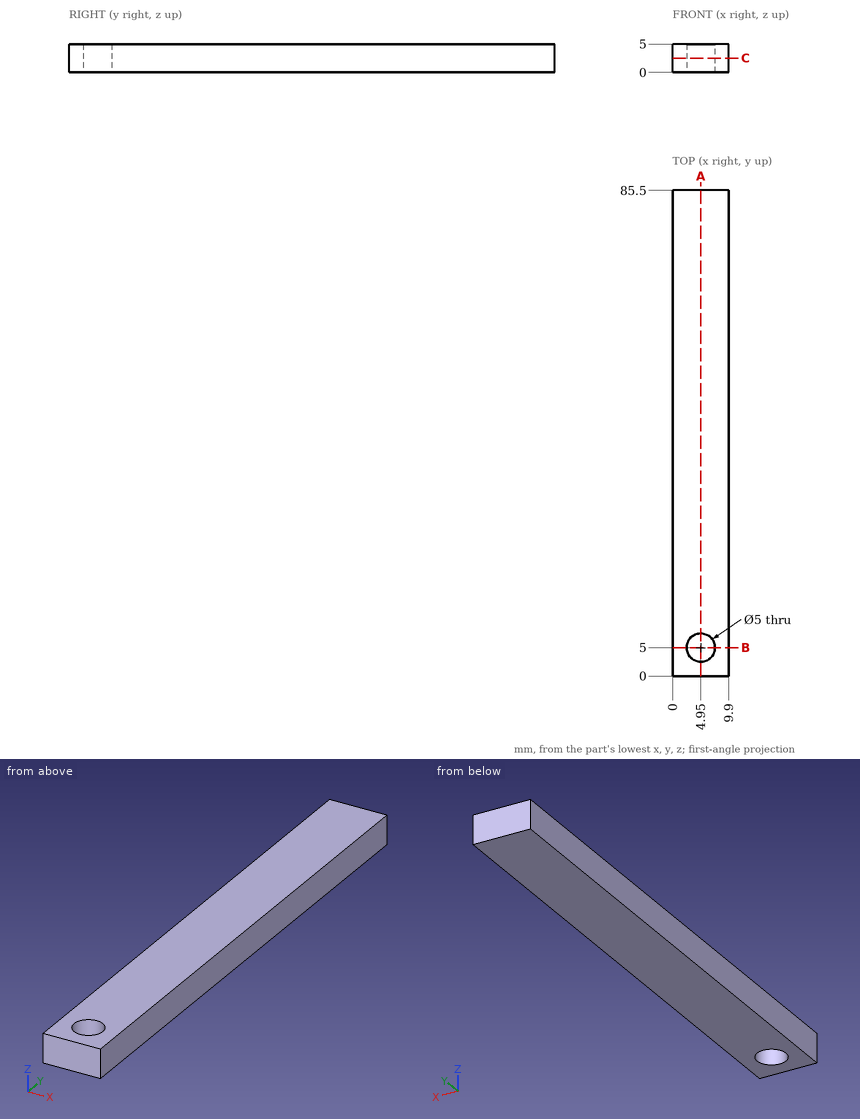
Geometry check sheet. Reference: drawing and pictorial views, mm from the part's lowest x, y, z. Round coordinates to 2 decimals unless told otherwise and drop trailing zeros. Order: outer loops, then holes, each group sorted by start corner. A loop starts at its lowest first (then second) coordinate and runs counter-clockwise, first axis right, second up. Notation, with made-up numbers: (82, 1.25) -> (121, 1.25) arc R17 ccw to (121, 5.25) -> close; hole circle Ø8 at (-39.5, 27.5). An arc over 180 degrees is marked (long way). One line per item, written item: value. Start each with the question number.
Q1. Cross-section at C-C (z = 2.5). Record the boundary of the cut face in (x, y).
Q2. Gauge pin test, flat end, axial feed: pin 1 Ø4 at (x, y) = (4.95, 5) entering from +Z. Record the tip position at first contact, or that the pin passes through.
Q3. Cross-section at A-A (x = 4.95). Record the boundary of the cut face in (y, z), and give its area (4 significant figures).
Q4. Cross-section at B-B (y = 5). Record the boundary of the cut face in (x, z), and give its area (3 significant figures).
Q5. Thickness scan on line 1 (X direction, y = 5, z = 2.1); line 2 (Y direction, x = 4.95, z = 3.5); line 3 (Y direction, x = 7, z = 2.15). Record the ranges inside material, lowest first.
Completed:
1. outline: (0, 0) -> (9.9, 0) -> (9.9, 85.5) -> (0, 85.5) -> close; hole circle Ø5 at (4.95, 5)
2. pin 1: passes through
3. outline: (0, 0) -> (2.5, 0) -> (2.5, 5) -> (0, 5) -> close; (7.5, 0) -> (85.5, 0) -> (85.5, 5) -> (7.5, 5) -> close
3. area: 402.5 mm²
4. outline: (0, 0) -> (2.45, 0) -> (2.45, 5) -> (0, 5) -> close; (7.45, 0) -> (9.9, 0) -> (9.9, 5) -> (7.45, 5) -> close
4. area: 24.5 mm²
5. line 1: x = 0 to 2.45, 7.45 to 9.9
5. line 2: y = 0 to 2.5, 7.5 to 85.5
5. line 3: y = 0 to 3.57, 6.43 to 85.5
